Build history of the part. All positions in model axes, mm. Face numbers are marked on the shaded views. A direction names the side the tool comes from. Round coordinates to 2 decimals unless told otherwise and drop trailing zeros. Write each loop counter-clockwise with the first axis right and the second up, starting at its lowest first coordinate (ties: lowest second). Pieces come first, ordered by that corner, then holes.
1) Flat gauge pins, fed straight in: pin 1 (2 mm diameter, centred on x = -9, z = 70.5, fed in from -Y); pin 2 (6 mm diameter, centred on y = -19, z = 85.5, fed in from -X); pin 3 (2.5 mm diameter, centred on x = 2, y = 24.5, fed in from +Z); pin 4 (2 mm diameter, centred on x = 18.5, y = -14, fed in from +Z). Where does each tip first touch, or does it go through?
2) Saw through at C-C (y = 2). Write the cut outline in (x, z).
3) Saw through at A-A (z = 13.5). Write the cut outline in (x, y), plus the area to 3 significant figures.
4) Wall check: probe 1 along Y at (x, z) = (9, 11); probe 2 along Z at (x, y) = (-23, -55); probe 3 along Y at (x, z) = (0.5, 58.5). Give the ranges that are in metal, low to high.
5) Saw through at B-B (x = 4.5). Write the cut outline in (y, z).
6) Pull direction Y, two halves, no side cores. Call the marked faces 4, 5 and 6: +Y half, -Y half, draft (parallel to the pull), parting line (faces both ways), or undercut.
7) Which spindle directions (+Z, -Z, +X, -X, +Y, -Y) get a long thin tool onto all of the face, cutting with end or side? Do the marked faces 1, 2 and 3. Say none if no direction does.
8) Saw through at D-D (z = 37.5). Write the cut outline in (x, y).
from build123d import *

# Parameters (mm, degrees)
SKETCH6_W           = 55.461011284
SKETCH6_H           = 53
BOSS_EXTRUDE5_DEPTH = 3
SKETCH7_W           = 55.461011284
SKETCH7_H           = 3
BOSS_EXTRUDE6_DEPTH = 23
SKETCH8_W           = 55.461011284
SKETCH8_H           = 3
BOSS_EXTRUDE7_DEPTH = 150
SKETCH9_W           = 55.461011284
SKETCH9_H           = 35
BOSS_EXTRUDE8_DEPTH = 3
FILLET2_R           = 10
FILLET3_R           = 10
FILLET5_R           = 5
FILLET6_R           = 5


with BuildPart() as part:
    # Sketch6 → Boss-Extrude5 (new body)
    with BuildSketch(Plane.XY):
        Rectangle(SKETCH6_W, SKETCH6_H)
    extrude(amount=BOSS_EXTRUDE5_DEPTH)

    # Sketch7 → Boss-Extrude6 (add)
    with BuildSketch(Plane.XY.offset(3)):
        with Locations((0, 25)):
            Rectangle(SKETCH7_W, SKETCH7_H)
        with Locations((0, -18)):
            Rectangle(SKETCH7_W, SKETCH7_H)
    extrude(amount=BOSS_EXTRUDE6_DEPTH)

    # Sketch8 → Boss-Extrude7 (add)
    with BuildSketch(Plane.XY.offset(3)):
        with Locations((0, -25)):
            Rectangle(SKETCH8_W, SKETCH8_H)
    extrude(amount=BOSS_EXTRUDE7_DEPTH)

    # Sketch9 → Boss-Extrude8 (add)
    with BuildSketch(Plane.XY.offset(153)):
        with Locations((0, -41)):
            Rectangle(SKETCH9_W, SKETCH9_H)
    extrude(amount=BOSS_EXTRUDE8_DEPTH)

    # Fillet2
    fillet2_edges = [part.edges().sort_by_distance(p)[0] for p in [
        (0, -26.5, 153),
    ]]
    fillet(fillet2_edges, radius=FILLET2_R)

    # Fillet3
    fillet3_edges = [part.edges().sort_by_distance(p)[0] for p in [
        (0, -23.5, 156),
    ]]
    fillet(fillet3_edges, radius=FILLET3_R)

    # Fillet5
    fillet5_edges = [part.edges().sort_by_distance(p)[0] for p in [
        (0, -26.5, 0),
    ]]
    fillet(fillet5_edges, radius=FILLET5_R)

    # Fillet6
    # the kernel refuses this fillet: 5 mm, written as the material it adds along each edge
    with BuildSketch(Plane(origin=(-27.730505642, -23.5, 3), x_dir=(0, 0, 1), z_dir=(1, 0, 0))) as fillet6_piece_1:
        with BuildLine():
            CenterArc((4.898979486, -5), FILLET6_R, 90, 78.463040967)
            Line((0, -4), (-0.09797959, -3.98))
            ThreePointArc((-0.09797959, -3.98), (-0.1, -2), (-0.1, 0))
            Line((-0.1, 0), (0, 0.1))
            Line((0, 0.1), (4.898979486, 0.1))
            Line((4.898979486, 0.1), (4.898979486, 0))
        make_face()
    extrude(amount=55.461011285)


solid = part.part
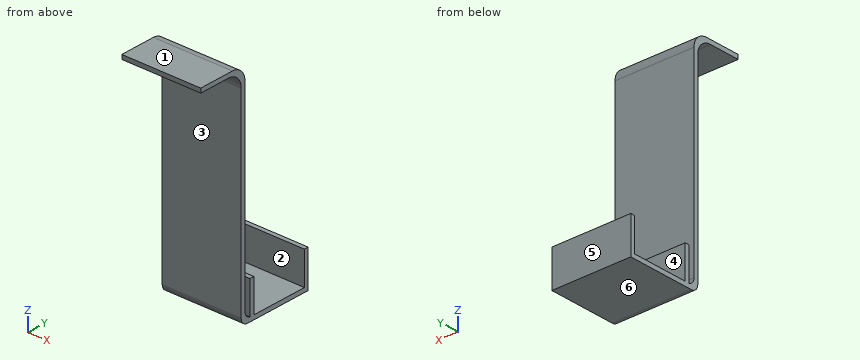
Evaluation:
1. pin 1: stops at y = -26.5
1. pin 2: passes through
1. pin 3: stops at z = 26
1. pin 4: stops at z = 3
2. outline: (-27.73, 0) - (27.73, 0) - (27.73, 3) - (-27.73, 3) - close
3. outline: (-27.73, -26.5) - (27.73, -26.5) - (27.73, -23.5) - (-27.73, -23.5) - close; (-27.73, -19.5) - (27.73, -19.5) - (27.73, -16.5) - (-27.73, -16.5) - close; (-27.73, 23.5) - (27.73, 23.5) - (27.73, 26.5) - (-27.73, 26.5) - close
3. area: 499 mm2
4. probe 1: y = -26.5 to -23.5, -19.5 to -16.5, 23.5 to 26.5
4. probe 2: z = 153 to 156
4. probe 3: y = -26.5 to -23.5
5. outline: (-58.5, 153) - (-36.5, 153) arc R10 cw to (-26.5, 143) - (-26.5, 5) arc R5 ccw to (-21.5, 0) - (26.5, 0) - (26.5, 26) - (23.5, 26) - (23.5, 3) - (-16.5, 3) - (-16.5, 26) - (-19.5, 26) - (-19.5, 3) arc R5 cw to (-23.5, 7.9) - (-23.5, 146) arc R10 ccw to (-33.5, 156) - (-58.5, 156) - close
6. face 4: undercut
6. face 5: +Y half
6. face 6: draft
7. face 1: +Z, +X, -X, +Y, -Y
7. face 2: +Z, +X, -X
7. face 3: -Z, +X, -X, -Y
8. outline: (-27.73, -26.5) - (27.73, -26.5) - (27.73, -23.5) - (-27.73, -23.5) - close
